Geometry check sheet. Reference: the model listing, model coordinates, mm. Face numbers are marked on the shaded views. A direction names the side the tool comes from. Give positions to 0.01 mm unless a question says otherwise; leave off trailing zeros. Loops run counter-clockwise (first coordinate to the right, second up) from the corner with the lowest first, then second, coordinate; pieces in that order, holes last. Notation, with made-up numbers: (-3, 59) -> (44, 59) arc R15 ccw to (44, 85) -> close; hole circle Ø8 at (58, 59). An arc over 180 degrees is marked (long way). Write item = value, one per line. Start each with the question number.
```python
from build123d import *

# Parameters (mm, degrees)
SKETCH1_R              = 9.525
BOSS_EXTRUDE1_DEPTH    = 3
SKETCH3_W              = 6
SKETCH3_H              = 12.7
BOSS_EXTRUDE2_DEPTH    = 6
FILLET1_R              = 1.27
LPATTERN1_COUNT        = 2
LPATTERN1_PITCH        = 25.4
FILLET1_OF_LPATTERN1_R = 1.27


with BuildPart() as part:
    # Sketch1 → Boss-Extrude1 (new, symmetric)
    with BuildSketch(Plane(origin=(0, 0, 0), x_dir=(0, 0, -1), z_dir=(1, 0, 0))):
        with BuildLine():
            Line((-15.540953853, 3.23950279), (-9.525, 32.1))
            Line((-9.525, 32.1), (34.925, 32.1))
            Line((34.925, 32.1), (14.034766421, -7.41895926))
            ThreePointArc((14.034766421, -7.41895926), (-5.382179248, -14.934783947), (-15.540953853, 3.23950279))
        make_face()
        Circle(SKETCH1_R, mode=Mode.SUBTRACT)
    extrude(amount=BOSS_EXTRUDE1_DEPTH, both=True)

    # Sketch3 → Boss-Extrude2 (add)
    with BuildSketch(Plane(origin=(0, 32.1, 0), x_dir=(1, 0, 0), z_dir=(0, 1, 0))):
        Rectangle(SKETCH3_W, SKETCH3_H)
    boss_extrude2 = extrude(amount=BOSS_EXTRUDE2_DEPTH)

    # Fillet1
    fillet1_edges = [part.edges().sort_by_distance(p)[0] for p in [
        (0, 38.1, -6.35),
        (0, 38.1, 6.35),
    ]]
    fillet(fillet1_edges, radius=FILLET1_R)

    # LPattern1: Boss-Extrude2 ×2
    with Locations(*[(0, 0, -i * LPATTERN1_PITCH) for i in range(1, LPATTERN1_COUNT)]):
        add(boss_extrude2)

    # Fillet1 of LPattern1
    fillet1_of_lpattern1_edges = [part.edges().sort_by_distance(p)[0] for p in [
        (0, 38.1, -31.75),
        (0, 38.1, -19.05),
    ]]
    fillet(fillet1_of_lpattern1_edges, radius=FILLET1_OF_LPATTERN1_R)


solid = part.part
```
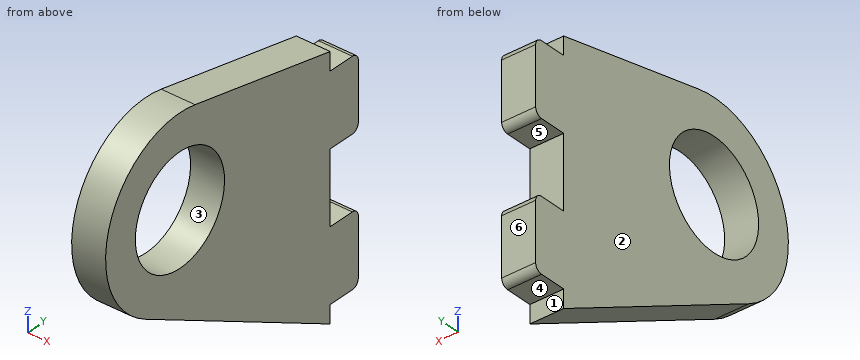
1) Section check A-A (z = 0). Enter the section's corners in (x, y) (3 decimals), plus the area to 3 significant figures.
2) Tool access check on the marked faces 4, 5 and 6. Record the directions out of +Z, -Z, +X, -X, +Y, -Y that give a thin tool (end or side, any length) a straight path to the whole face; none if there is none.
3) Section check C-C (y = 5.5). Enter the section's corners in (x, z).
4) Thickness scan on line 1 (Y direction, x = -0.6, z = 0) (3 decimals); line 2 (Y direction, x = -0.8, z = 8); line 3 (Z direction, x = -0.2, y = 6.5). Record the ranges inside material, lowest first.
5) Draft check along Y on the marked faces 1, 2 and 3. Enter one of: released by +Y, released by -Y, zero draft, split by the parting line, or undercut.
6) Depth check by flat-ended pin: pin 1 Ø1.4 at (x, y) = (-1, 34.5) entering from -Z; pin 2 Ø1.5 at (x, z) = (-2, -29) entering from -Y; pin 3 Ø1.5 at (x, z) = (1, -10.5) entering from -Y. Enter the tip coordinate at first touch or a pass-through.
7) Section check D-D (y = 14.5). Enter the section's corners in (x, z).
Check result:
q1.outline = (-3, -15.875) -> (3, -15.875) -> (3, -9.525) -> (-3, -9.525) -> close; (-3, 9.525) -> (3, 9.525) -> (3, 38.1) -> (-3, 38.1) -> close
q1.area = 210 mm2
q2.face_4 = -Z, +X, -X, +Y
q2.face_5 = +X, -X, +Y
q2.face_6 = +Z, -Z, +X, -X, +Y
q3.outline = (-3, -20.86) -> (3, -20.86) -> (3, -7.78) -> (-3, -7.78) -> close; (-3, 7.78) -> (3, 7.78) -> (3, 15.07) -> (-3, 15.07) -> close
q4.line_1 = -15.875 to -9.525, 9.525 to 38.1
q4.line_2 = -13.71 to -5.17, 5.17 to 32.1
q4.line_3 = -21.39 to -6.96, 6.96 to 14.86
q5.face_1 = released by +Y
q5.face_2 = zero draft
q5.face_3 = undercut
q6.pin_1 = -31.75
q6.pin_2 = 19.47
q6.pin_3 = -12.53
q7.outline = (-3, -25.62) -> (3, -25.62) -> (3, 13.19) -> (-3, 13.19) -> close
